from build123d import *

# Parameters (mm, degrees)
BOSS_EXTRU_1_DEPTH                                   = 470
ESQUISSE2_R                                          = 1.15
ESQUISSE2_R_2                                        = 1.6
ENL_V_MAT_EXTRU_1_DEPTH                              = 471.395843944
TROU_POUR_TARAUDAGE_POUR_TROU_TARAUD_M3_D            = 2.5
FORMSENKUNG_F_R_M2_SENKSCHRAUBE_MIT_SCHL_D           = 2.4
FORMSENKUNG_F_R_M2_SENKSCHRAUBE_MIT_SCHL_DEPTH       = 5
FORMSENKUNG_F_R_M2_SENKSCHRAUBE_MIT_SCHL_CSINK_D     = 4.4
FORMSENKUNG_F_R_M2_SENKSCHRAUBE_MIT_SCHL_CSINK_ANGLE = 90
FORMSENKUNG_F_R_M2_SENKSCHRAUBE_MIT_SCHL_TIP         = 0.721032743
FORMSENKUNG_F_R_M2_SENKSCHRAUBE_MIT_2_D              = 2.4
FORMSENKUNG_F_R_M2_SENKSCHRAUBE_MIT_2_DEPTH          = 5
FORMSENKUNG_F_R_M2_SENKSCHRAUBE_MIT_2_CSINK_D        = 4.4
FORMSENKUNG_F_R_M2_SENKSCHRAUBE_MIT_2_CSINK_ANGLE    = 90
FORMSENKUNG_F_R_M2_SENKSCHRAUBE_MIT_2_TIP            = 0.721032743
FORMSENKUNG_F_R_M3_SENKSCHRAUBE_MIT_SCHL_D           = 3.4
FORMSENKUNG_F_R_M3_SENKSCHRAUBE_MIT_SCHL_DEPTH       = 5
FORMSENKUNG_F_R_M3_SENKSCHRAUBE_MIT_SCHL_CSINK_D     = 6.3
FORMSENKUNG_F_R_M3_SENKSCHRAUBE_MIT_SCHL_CSINK_ANGLE = 90
FORMSENKUNG_F_R_M3_SENKSCHRAUBE_MIT_SCHL_TIP         = 1.021463052
FORMSENKUNG_F_R_M3_SENKSCHRAUBE_MIT_2_D              = 3.4
FORMSENKUNG_F_R_M3_SENKSCHRAUBE_MIT_2_CSINK_D        = 6.3
FORMSENKUNG_F_R_M3_SENKSCHRAUBE_MIT_2_CSINK_ANGLE    = 90


with BuildPart() as part:
    # Esquisse1 → Boss.-Extru.1 (new body)
    with BuildSketch(Plane.XY):
        Polygon((-8.25, 0), (8.25, 0), (8.25, 10), (6.75, 10), (6.75, 2), (-6.75, 2), (-6.75, 10), (-8.25, 10), align=None)
    extrude(amount=BOSS_EXTRU_1_DEPTH)

    # Esquisse2 → Enlèv. mat.-Extru.1 (cut, through all)
    with BuildSketch(Plane(origin=(8.25, 0, 0), x_dir=(0, 0, -1), z_dir=(1, 0, 0))):
        with Locations((-440, 8)):
            Circle(ESQUISSE2_R)
        with Locations((-440, 3.5)):
            Circle(ESQUISSE2_R)
        with Locations((-430, 7)):
            Circle(ESQUISSE2_R_2)
    extrude(amount=-ENL_V_MAT_EXTRU_1_DEPTH, mode=Mode.SUBTRACT)

    # Trou pour taraudage pour trou taraudé M31 (through all)
    with Locations(Plane(origin=(0, 2, 0), x_dir=(1, 0, 0), z_dir=(0, 1, 0))):
        with Locations((0, -465)):
            Hole(TROU_POUR_TARAUDAGE_POUR_TROU_TARAUD_M3_D / 2)

    # Formsenkung f_r M2 Senkschraube mit Schl
    with Locations(Plane(origin=(8.25, 0, 0), x_dir=(0, 0, -1), z_dir=(1, 0, 0))):
        with Locations((-440, 3.5), (-440, 8)):
            CounterSinkHole(FORMSENKUNG_F_R_M2_SENKSCHRAUBE_MIT_SCHL_D / 2, FORMSENKUNG_F_R_M2_SENKSCHRAUBE_MIT_SCHL_CSINK_D / 2, depth=FORMSENKUNG_F_R_M2_SENKSCHRAUBE_MIT_SCHL_DEPTH, counter_sink_angle=FORMSENKUNG_F_R_M2_SENKSCHRAUBE_MIT_SCHL_CSINK_ANGLE)
            with Locations((0, 0, -(FORMSENKUNG_F_R_M2_SENKSCHRAUBE_MIT_SCHL_DEPTH + FORMSENKUNG_F_R_M2_SENKSCHRAUBE_MIT_SCHL_TIP / 2))):  # 118° drill point
                Cone(0, FORMSENKUNG_F_R_M2_SENKSCHRAUBE_MIT_SCHL_D / 2, FORMSENKUNG_F_R_M2_SENKSCHRAUBE_MIT_SCHL_TIP, mode=Mode.SUBTRACT)

    # Formsenkung f_r M2 Senkschraube mit  2
    with Locations(Plane.ZY.offset(8.25)):
        with Locations((440, 8), (440, 3.5)):
            CounterSinkHole(FORMSENKUNG_F_R_M2_SENKSCHRAUBE_MIT_2_D / 2, FORMSENKUNG_F_R_M2_SENKSCHRAUBE_MIT_2_CSINK_D / 2, depth=FORMSENKUNG_F_R_M2_SENKSCHRAUBE_MIT_2_DEPTH, counter_sink_angle=FORMSENKUNG_F_R_M2_SENKSCHRAUBE_MIT_2_CSINK_ANGLE)
            with Locations((0, 0, -(FORMSENKUNG_F_R_M2_SENKSCHRAUBE_MIT_2_DEPTH + FORMSENKUNG_F_R_M2_SENKSCHRAUBE_MIT_2_TIP / 2))):  # 118° drill point
                Cone(0, FORMSENKUNG_F_R_M2_SENKSCHRAUBE_MIT_2_D / 2, FORMSENKUNG_F_R_M2_SENKSCHRAUBE_MIT_2_TIP, mode=Mode.SUBTRACT)

    # Formsenkung f_r M3 Senkschraube mit Schl
    with Locations(Plane(origin=(8.25, 0, 0), x_dir=(0, 0, -1), z_dir=(1, 0, 0))):
        with Locations((-430, 7)):
            CounterSinkHole(FORMSENKUNG_F_R_M3_SENKSCHRAUBE_MIT_SCHL_D / 2, FORMSENKUNG_F_R_M3_SENKSCHRAUBE_MIT_SCHL_CSINK_D / 2, depth=FORMSENKUNG_F_R_M3_SENKSCHRAUBE_MIT_SCHL_DEPTH, counter_sink_angle=FORMSENKUNG_F_R_M3_SENKSCHRAUBE_MIT_SCHL_CSINK_ANGLE)
            with Locations((0, 0, -(FORMSENKUNG_F_R_M3_SENKSCHRAUBE_MIT_SCHL_DEPTH + FORMSENKUNG_F_R_M3_SENKSCHRAUBE_MIT_SCHL_TIP / 2))):  # 118° drill point
                Cone(0, FORMSENKUNG_F_R_M3_SENKSCHRAUBE_MIT_SCHL_D / 2, FORMSENKUNG_F_R_M3_SENKSCHRAUBE_MIT_SCHL_TIP, mode=Mode.SUBTRACT)

    # Formsenkung f_r M3 Senkschraube mit  2 (through all)
    with Locations(Plane(origin=(-8.25, -1.5, 0), x_dir=(0, 0, -1), z_dir=(-1, 0, 0))):
        with Locations((-100, -6.5)):
            CounterSinkHole(FORMSENKUNG_F_R_M3_SENKSCHRAUBE_MIT_2_D / 2, FORMSENKUNG_F_R_M3_SENKSCHRAUBE_MIT_2_CSINK_D / 2, counter_sink_angle=FORMSENKUNG_F_R_M3_SENKSCHRAUBE_MIT_2_CSINK_ANGLE)


solid = part.part
Geometry: final body of the model. Coordinates: model frame, mm. A direction names the side the tool comes from. Give positions to 0.01 mm unless a question says otherwise; leave off trailing zeros. Order: outer loops, then holes, each group sorted by start corner. A loop starts at its lowest first (then second) coordinate and runs counter-clockwise, first axis right, second up. Notation, with made-up numbers: (70.5, 18) -> (77.5, 18) arc R27 ccw to (77.5, 57) -> close; hole circle Ø6 at (-31.5, 17). An arc over 180 degrees is marked (long way). Write each question's results on one line, items separated by ' | '.
1) Cut plane A-A (z = 373). Output: boundary loops of the cut face in (x, y).
Geometry says:
outline: (-8.25, 0) -> (8.25, 0) -> (8.25, 10) -> (6.75, 10) -> (6.75, 2) -> (-6.75, 2) -> (-6.75, 10) -> (-8.25, 10) -> close
2) Set-up query: faces 4 (the face through (-6.75, 6, 232)), 5 (the face through (-0.1, 1.7, 470)). Return all of +Z, -Z, +X, -X, +Y, -Y with unobstructed straight access to the full face (end or side cutting, diameter ignored); none if empty.
Geometry says:
face 4: +Z, -Z, +Y | face 5: +Z, +X, -X, +Y, -Y
3) Draft query along X for faces 1 (the face through (-0.1, 1.7, 0)), 2 (the face through (-8.25, 5, 232)), 3 (the face through (6.75, 6, 232)). Return one class per face: released by +X, released by -X, zero draft, split by the parting line, or undercut.
Geometry says:
face 1: zero draft | face 2: released by -X | face 3: undercut
4) Line query: line 1 along Y through (x, z) = (7.05, 440); line 2 along X through (y, z) = (4.5, 244.5); line 3 along Y through (x, z) = (7.45, 100). Output: solid intervals per line, ascending.
Geometry says:
line 1: y = 0 to 2.3, 4.7 to 6.8, 9.2 to 10 | line 2: x = -8.25 to -6.75, 6.75 to 8.25 | line 3: y = 0 to 3.3, 6.7 to 10
5) First-contact query: pin 1 Ø3 at (y, z) = (8, 440) entering from +X; pin 2 Ø5.5 at (y, z) = (7, 430) entering from +X. Flat tips, straight axial feed; report the tip coordinate or a pass-through.
Geometry says:
pin 1: stops at x = 7.55 | pin 2: stops at x = 7.85
